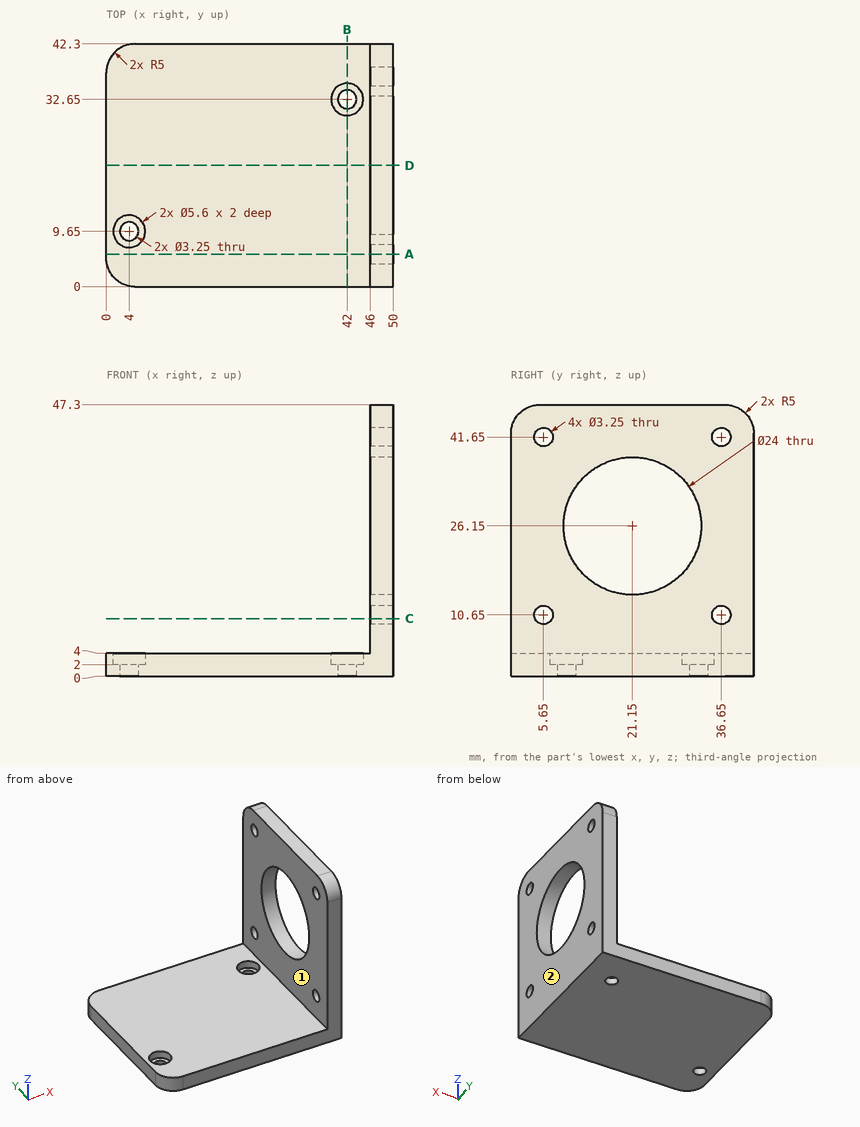
Geometry check sheet. Reference: drawing and pictorial views, mm from the part's lowest x, y, z. A direction names the side the tool comes from. Round coordinates to 2 decimals unless told otherwise and drop trailing zeros. Loops run counter-clockwise (first coordinate to the right, second up) from the corner with the lowest first, then second, coordinate; pieces in that order, holes last. Notation, with made-up numbers: (58.5, -37.5) - (105.5, -37.5) arc R27 ccw to (105.5, -10.5) - close; hole circle Ø2 at (3.25, -4.5). An arc over 180 degrees is marked (long way). One line per question, with ' | ' between items. Start each with the question number.
1. Depth check by flat-ended pin: pin 1 (3.5 mm diameter, centred on y = 5.65, z = 10.65, fed in from -X); pin 2 (3 mm diameter, centred on x = 17, y = 4.5, fed in from +Z); pin 3 (5 mm diameter, centred on x = 42, y = 32.65, fed in from +Z). Enter the tip coordinate at first touch or a pass-through.
2. Cross-section at D-D on y = 21.15. Record the cut outline in (x, z).
3. Scan lines: line 1 (Z direction, x = 47, y = 5.65) (3 decimals); line 2 (Y direction, x = 47, z = 41); line 3 (X direction, y = 32.5, z = 31.5). Record each from-to range of solid material in increasing order. Write a range as [from, to].
4. Tool access check on the marked faces 1 and 2. Record the directions out of +Z, -Z, +X, -X, +Y, -Y that give a thin tool (end or side, any length) a straight path to the whole face; none if there is none.
5. Cross-section at C-C on z = 10. Record the cut outline in (x, y).
6. Cross-section at B-B on x = 42. Record the cut outline in (y, z) (3 decimals).
7. Cross-section at A-A on y = 5.65. Record the cut outline in (x, z) (3 decimals).
Taken from the geometry:
1) pin 1: x = 46 | pin 2: z = 4 | pin 3: z = 2
2) outline: (0, 0) - (50, 0) - (50, 14.15) - (46, 14.15) - (46, 4) - (0, 4) - close; (46, 38.15) - (50, 38.15) - (50, 47.3) - (46, 47.3) - close
3) line 1: [0, 9.025], [12.275, 40.025], [43.275, 47.3] | line 2: [0, 4.16], [7.14, 35.16], [38.14, 42.3] | line 3: [46, 50]
4) face 1: +Z, -X, +Y, -Y | face 2: +Z, -Z, +X, +Y, -Y
5) outline: (46, 0) - (50, 0) - (50, 4.16) - (46, 4.16) - close; (46, 7.14) - (50, 7.14) - (50, 35.16) - (46, 35.16) - close; (46, 38.14) - (50, 38.14) - (50, 42.3) - (46, 42.3) - close
6) outline: (0, 0) - (31.025, 0) - (31.025, 2) - (29.85, 2) - (29.85, 4) - (0, 4) - close; (34.275, 0) - (42.3, 0) - (42.3, 4) - (35.45, 4) - (35.45, 2) - (34.275, 2) - close
7) outline: (0, 0) - (50, 0) - (50, 9.025) - (46, 9.025) - (46, 4) - (0, 4) - close; (46, 12.275) - (50, 12.275) - (50, 40.025) - (46, 40.025) - close; (46, 43.275) - (50, 43.275) - (50, 47.3) - (46, 47.3) - close
